from build123d import *

# Parameters (mm, degrees)
SKETCH1_R                = 31.7
SKETCH1_R_2              = 29.7
BOSS_EXTRUDE1_DEPTH      = 200
BOSS_EXTRUDE2_DEPTH      = 63
BOSS_EXTRUDE3_DEPTH      = 5.5
BOSS_EXTRUDE3_DEPTH_BACK = 23


with BuildPart() as part:
    # Sketch1 → Boss-Extrude1 (new body)
    with BuildSketch(Plane.XY):
        Circle(SKETCH1_R)
        Circle(SKETCH1_R_2, mode=Mode.SUBTRACT)
    extrude(amount=BOSS_EXTRUDE1_DEPTH)

    # Sketch4 → Boss-Extrude2 (add)
    with BuildSketch(Plane(origin=(0, 0, 100), x_dir=(-1, 0, 0), z_dir=(0, 0, -1))):
        with BuildLine():
            Line((-6.85, 32.897074338), (-6.85, 58.2))
            Line((-6.85, 58.2), (6.85, 58.2))
            Line((6.85, 58.2), (6.85, 32.897074338))
            ThreePointArc((6.85, 32.897074338), (7.355169327, 31.390206532), (8.666520468, 30.492317442))
            ThreePointArc((8.666520468, 30.492317442), (12.352096929, 29.194446415), (15.85, 27.4530053))
            Line((15.85, 27.4530053), (16.8, 29.098453567))
            ThreePointArc((16.8, 29.098453567), (13.092443432, 30.944271279), (9.185964912, 32.319932683))
            ThreePointArc((9.185964912, 32.319932683), (8.871240638, 32.535426065), (8.75, 32.897074338))
            Line((8.75, 32.897074338), (8.75, 58.2))
            ThreePointArc((8.75, 58.2), (8.193502884, 59.543502884), (6.85, 60.1))
            Line((6.85, 60.1), (-6.85, 60.1))
            ThreePointArc((-6.85, 60.1), (-8.193502884, 59.543502884), (-8.75, 58.2))
            Line((-8.75, 58.2), (-8.75, 32.897074338))
            ThreePointArc((-8.75, 32.897074338), (-8.871240638, 32.535426065), (-9.185964912, 32.319932683))
            ThreePointArc((-9.185964912, 32.319932683), (-13.092443432, 30.944271279), (-16.8, 29.098453567))
            Line((-16.8, 29.098453567), (-15.85, 27.4530053))
            ThreePointArc((-15.85, 27.4530053), (-12.352096929, 29.194446415), (-8.666520468, 30.492317442))
            ThreePointArc((-8.666520468, 30.492317442), (-7.355169327, 31.390206532), (-6.85, 32.897074338))
        make_face()
    extrude(amount=BOSS_EXTRUDE2_DEPTH)

    # Sketch5 one side → Revolve1 (revolve)
    with BuildSketch(Plane.ZY):
        with BuildLine():
            Line((68.5, 60.1), (68.5, 65.1))
            ThreePointArc((68.5, 65.1), (64.964466094, 63.635533906), (63.5, 60.1))
            Line((63.5, 60.1), (68.5, 60.1))
        make_face()
    revolve(axis=Axis((0, 60.1, 68.5), (0, 1, 0)))

    # Sketch6 → Boss-Extrude3 (add, two sides)
    with BuildSketch(Plane.ZY.offset(8.75)) as boss_extrude3_sk:
        Polygon((72.25277675, 44.7), (76.005553499, 51.2), (72.25277675, 57.7), (64.74722325, 57.7), (60.994446501, 51.2), (64.74722325, 44.7), align=None)
    extrude(amount=BOSS_EXTRUDE3_DEPTH)
    extrude(boss_extrude3_sk.sketch, amount=-BOSS_EXTRUDE3_DEPTH_BACK)


solid = part.part
Source: CAD feature listing. Evaluate the final solid. Frame: model axes, mm. A direction names the side the tool comes from. Give positions to 0.01 mm unless a question says otherwise; leave off trailing zeros. Write each loop counter-clockwise with the first axis right and the second up, starting at its lowest first coordinate (ties: lowest second). Pieces come first, ordered by that corner, then holes. Notation, with made-up numbers: M 54,-32.75 L 81,-32.75 A14 cw 81,-8.75 Z; hole C -38.75,43 d4. An arc over 180 degrees is marked long. Answer as a JSON object with one key per item and string values.
Q1. Contact query for flat-ended pins moving along their axis: P1, Ø6.5, axis at y = 52.5, z = 70.5, coming from the -X side; P2, Ø1, axis at x = -22, z = 121.5, coming from the +Y side; P3, Ø10, axis at y = 26.5, z = 153.5, coming from the +X side; P4, Ø8, axis at x = 21, y = 7, coming from the +Z side. Output: stop coordinate, or through.
Geometry check:
{"P1": "stops at x = -14.25", "P2": "stops at y = 23.29", "P3": "stops at x = 23.29", "P4": "passes through"}
Q2. Cut plane D-D, the plane z = 142. Return the cut outline in (x, y), then the cut area to 3 significant figures.
Geometry check:
{"outline": "C 0,0 d63.4; hole C 0,0 d59.4", "area": "386 mm^2"}
Q3. Ray query, line 1 along Y through (x, z) = (0, 127.5); line 2 along Y through (x, z) = (-22, 128.5); line 3 along X through (y, z) = (3, 136). Return the intervals inside material, ascending.
Geometry check:
{"line 1": "y = -31.7 to -29.7, 29.7 to 31.7", "line 2": "y = -22.82 to -19.95, 19.95 to 22.82", "line 3": "x = -31.56 to -29.55, 29.55 to 31.56"}
Q4. Access query for faces 5 (the face through (-11.46, 48, 62.84)), 6 (the face through (-0.1, 48, 62.84)), 7 (the face through (-14.25, 51, 68)). Directions: +Z, -Z, +X, -X, +Y, -Y. A direction counts if a zero-diameter tool reaches every point of the face in a straight line with its end or side. Return the directions, or none.
Geometry check:
{"face 5": "-Z, -X", "face 6": "-Z", "face 7": "+Z, -Z, -X, +Y"}
Q5. Mould query, pull axis X, two halves, no side actions, for faces 1 (the face through (-0.1, 54.5, 62.9)), 2 (the face through (-11, 44.7, 68)), 3 (the face through (-13.15, 30.92, 68.94)), 4 (the face through (-6.85, 43, 69)). Classes: +X half, -X half, draft (parallel to the pull), parting line (faces both ways), or undercut.
Geometry check:
{"face 1": "undercut", "face 2": "draft", "face 3": "-X half", "face 4": "undercut"}
Q6. Cut plane C-C, the plane x = 26. Return the cut outline in (y, z).
Geometry check:
{"outline": "M -18.14,0 L -14.36,0 L -14.36,200 L -18.14,200 Z; M 14.36,0 L 18.14,0 L 18.14,200 L 14.36,200 Z"}
Q7. Cut plane B-B, the plane y = 0. Return the cut outline in (x, z).
Geometry check:
{"outline": "M -31.7,0 L -29.7,0 L -29.7,200 L -31.7,200 Z; M 29.7,0 L 31.7,0 L 31.7,200 L 29.7,200 Z"}
Q8. Cut plane A-A, the plane x = 0. Return the cut outline in (y, z).
Geometry check:
{"outline": "M -31.7,0 L -29.7,0 L -29.7,200 L -31.7,200 Z; M 29.7,0 L 31.7,0 L 31.7,200 L 29.7,200 Z; M 44.7,64.75 L 51.2,60.99 L 57.7,64.75 L 57.7,72.25 L 51.2,76.01 L 44.7,72.25 Z; M 58.2,37 L 60.1,37 L 60.1,63.5 A5 ccw 60.1,73.5 L 60.1,100 L 58.2,100 Z"}
